Answer from the drawing. Dimensions are ordinates in mm from the lowest x, y and z of the part. Coordinates: 2 decimals unless noted, no trailing zeros. Write each loop counter-clockwise with the first axis right and the second up, starting at its lowest first coordinate (ties: lowest second). Pieces come first, ordered by that corner, then holes. Notation, with made-up numbers: (79, -10) -> (89, -10) arc R34 cw to (89, 28) -> close; hole circle Ø7 at (-12, -1.5). An arc over 180 degrees is marked (long way). Answer as a JSON object with one key per item and string values. Group by question number.
(1) Find section C-C (y = 95). Give the vertices of the cut face in (x, z), then the cut area to 3 significant figures.
(2) Flat-ended cylindrical pins translate along their axes: P1, Ø0.9, axis at y = 54, z = 2, coming from the -X side; P2, Ø3.5, axis at x = 35, y = 5, coming from the +Z side; P3, Ø1, axis at x = 15, z = 2, coming from the -Y side; P4, Ø1.5, axis at y = 27, z = 1, coming from the -X side. Find the tip coordinate at first contact, or state that the pin passes through.
(3) Find section A-A (x = 5). Give the vertices of the cut face in (y, z), then the cut area to 3 significant figures.
(4) Find section B-B (y = 14). Give the vertices of the cut face in (x, z).
(5) Straight lines are drawn through the part: L1, parallel to Y at x = 35, z = 2.2; L2, parallel to Y at x = 5, z = 2.1; L3, parallel to X at y = 95, z = 1.6. For each, find the intervals that lie inside material, in ascending order.
(6) Find section D-D (x = 15). Give the vertices of the cut face in (y, z).
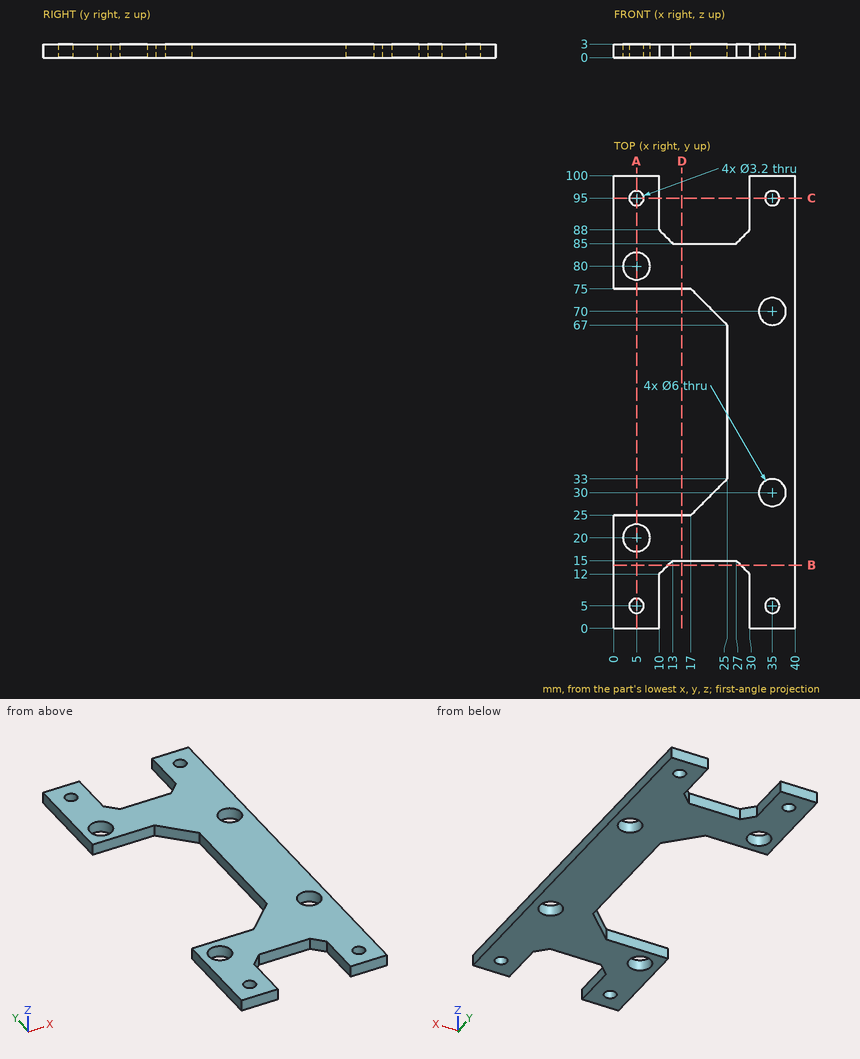
Results below:
{
 "1": {"outline": "(0, 0) -> (3.4, 0) -> (3.4, 3) -> (0, 3) -> close; (6.6, 0) -> (10, 0) -> (10, 3) -> (6.6, 3) -> close; (30, 0) -> (33.4, 0) -> (33.4, 3) -> (30, 3) -> close; (36.6, 0) -> (40, 0) -> (40, 3) -> (36.6, 3) -> close", "area": "40.8 mm2"},
 "2": {"P1": "stops at x = 25", "P2": "stops at z = 3", "P3": "stops at y = 15", "P4": "stops at x = 18.25"},
 "3": {"outline": "(0, 0) -> (3.4, 0) -> (3.4, 3) -> (0, 3) -> close; (6.6, 0) -> (17, 0) -> (17, 3) -> (6.6, 3) -> close; (23, 0) -> (25, 0) -> (25, 3) -> (23, 3) -> close; (75, 0) -> (77, 0) -> (77, 3) -> (75, 3) -> close; (83, 0) -> (93.4, 0) -> (93.4, 3) -> (83, 3) -> close; (96.6, 0) -> (100, 0) -> (100, 3) -> (96.6, 3) -> close", "area": "94.8 mm2"},
 "4": {"outline": "(0, 0) -> (12, 0) -> (12, 3) -> (0, 3) -> close; (28, 0) -> (40, 0) -> (40, 3) -> (28, 3) -> close"},
 "5": {"L1": "y = 0 to 3.4, 6.6 to 27, 33 to 67, 73 to 93.4, 96.6 to 100", "L2": "y = 0 to 3.4, 6.6 to 17, 23 to 25, 75 to 77, 83 to 93.4, 96.6 to 100", "L3": "x = 0 to 3.4, 6.6 to 10, 30 to 33.4, 36.6 to 40"},
 "6": {"outline": "(15, 0) -> (25, 0) -> (25, 3) -> (15, 3) -> close; (75, 0) -> (85, 0) -> (85, 3) -> (75, 3) -> close"}
}
